from build123d import *

# Parameters (mm, degrees)
SKETCH2_R           = 55
BOSS_EXTRUDE1_DEPTH = 70
SHELL1_T            = -5
SKETCH4_R           = 125
BOSS_EXTRUDE2_DEPTH = 1
RIB7_REACH          = 192.132
SKETCH3_WALL_W      = 472.644862012
SKETCH3_WALL_H      = 10
CIRPATTERN1_COUNT   = 4
CUT_EXTRUDE1_DEPTH  = 1
CIRPATTERN2_COUNT   = 4
CUT_EXTRUDE2_DEPTH  = 194.455421222
CIRPATTERN3_COUNT   = 4
SKETCH10_W          = 64.387061578
SKETCH10_H          = 55
CUT_EXTRUDE3_DEPTH  = 191.131533418
CIRPATTERN4_COUNT   = 2
CIRPATTERN4_ANGLE   = 90


with BuildPart() as part:
    # Sketch2 → Boss-Extrude1 (new body)
    with BuildSketch(Plane(origin=(0, 0, 0), x_dir=(1, 0, 0), z_dir=(0, 1, 0))):
        with Locations(Location((0, 0, 0), (0, 0, 270))):
            Circle(SKETCH2_R)
    extrude(amount=BOSS_EXTRUDE1_DEPTH)

    # Shell1
    shell1_openings = [part.faces().sort_by_distance(p)[0] for p in [
        (0, 70, 0),
    ]]
    offset(amount=SHELL1_T, openings=shell1_openings, kind=Kind.INTERSECTION)

    # Sketch4 → Boss-Extrude2 (add)
    with BuildSketch(Plane(origin=(0, 0, 0), x_dir=(1, 0, 0), z_dir=(0, 1, 0))):
        with Locations(Location((0, 0, 0), (0, 0, 270))):
            Circle(SKETCH4_R)
    extrude(amount=BOSS_EXTRUDE2_DEPTH)

    # Sketch3 wall → Rib7 (add, up to next)
    with BuildSketch(Plane(origin=(87, 32.90951621, 0), x_dir=(0.708107200971, -0.706104943994, 0), z_dir=(0.706104943994, 0.708107200971, 0)), mode=Mode.PRIVATE) as rib7_sk1:
        Rectangle(SKETCH3_WALL_W, SKETCH3_WALL_H)
    rib7_tool1 = extrude(rib7_sk1.sketch, amount=-RIB7_REACH, mode=Mode.PRIVATE) - part.part
    rib7 = rib7_tool1.solids().sort_by_distance((87, 32.90951621, 0))[0]
    add(rib7)

    # CirPattern1: Rib7 ×4 about axis
    cirpattern1_axis = Axis((0, 0, 0), (0, 1, 0))
    for i in range(1, CIRPATTERN1_COUNT):
        add(rib7.rotate(cirpattern1_axis, i * 360 / CIRPATTERN1_COUNT))

    # Sketch5 → Cut-Extrude1 (cut)
    with BuildSketch(Plane(origin=(0, 1, 0), x_dir=(1, 0, 0), z_dir=(0, 1, 0))):
        with BuildLine():
            Line((9.493142678, -59.24424227), (9.493142678, -129.652922227))
            ThreePointArc((9.493142678, -129.652922227), (92.201319164, -91.645604065), (129.707942461, -8.709171177))
            Line((129.707942461, -8.709171177), (59.364554554, -8.709171177))
            ThreePointArc((59.364554554, -8.709171177), (42.705900876, -42.145059383), (9.493142678, -59.24424227))
        make_face()
    cut_extrude1 = extrude(amount=-CUT_EXTRUDE1_DEPTH, mode=Mode.SUBTRACT)

    # CirPattern2: Cut-Extrude1 ×4 about axis
    cirpattern2_axis = Axis((0, 0, 0), (0, 1, 0))
    for i in range(1, CIRPATTERN2_COUNT):
        add(cut_extrude1.rotate(cirpattern2_axis, i * 360 / CIRPATTERN2_COUNT), mode=Mode.SUBTRACT)

    # Sketch7 → Cut-Extrude2 (cut, through all)
    with BuildSketch(Plane(origin=(5, 0, 0), x_dir=(0, 0, -1), z_dir=(1, 0, 0))):
        Polygon((59.772255751, 52.99919304), (106.904721419, 6), (59.772255751, 6), align=None)
    cut_extrude2 = extrude(amount=-CUT_EXTRUDE2_DEPTH, mode=Mode.SUBTRACT)

    # CirPattern3: Cut-Extrude2 ×4 about axis
    cirpattern3_axis = Axis((0, 0, 0), (0, 1, 0))
    for i in range(1, CIRPATTERN3_COUNT):
        add(cut_extrude2.rotate(cirpattern3_axis, i * 360 / CIRPATTERN3_COUNT), mode=Mode.SUBTRACT)

    # Sketch10 → Cut-Extrude3 (cut, symmetric)
    with BuildSketch(Plane(origin=(0, 0, 0), x_dir=(0.7117650145966598, -3.2873850610052313e-15, 0.7024176563813135), z_dir=(-0.7024176563813135, -3.331131634682351e-15, 0.7117650145966598))):
        with Locations((-0.279356343, 36.5)):
            Rectangle(SKETCH10_W, SKETCH10_H)
    cut_extrude3 = extrude(amount=CUT_EXTRUDE3_DEPTH, both=True, mode=Mode.SUBTRACT)

    # CirPattern4: Cut-Extrude3 ×2 about axis
    cirpattern4_axis = Axis((0, 70, 0), (0, 1, 0))
    for i in range(1, CIRPATTERN4_COUNT):
        add(cut_extrude3.rotate(cirpattern4_axis, i * CIRPATTERN4_ANGLE / (CIRPATTERN4_COUNT - 1)), mode=Mode.SUBTRACT)


solid = part.part
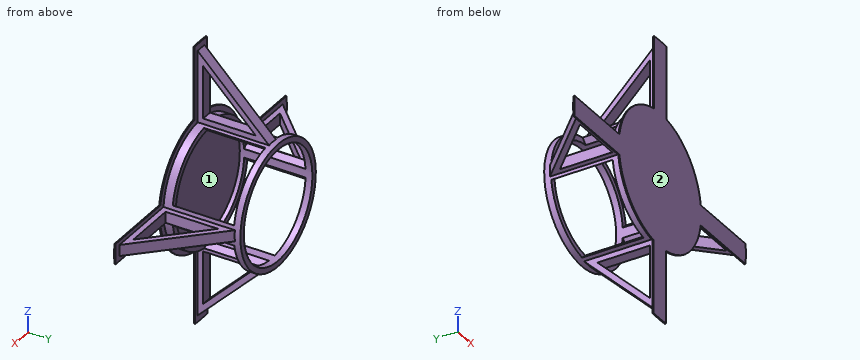
Input: part model. Units: mm. Frame: model coordinates. Face numbers are marked on the shaded views. Coordinates: 2 decimals unless noted, no trailing zeros. Loops run counter-clockwise (first coordinate to the right, second up) from the corner with the lowest first, then second, coordinate; pieces in that order, holes last. Notation, with made-up numbers: (-20.5, -31.5) -> (11.5, -31.5) arc R33 cw to (11.5, 4.5) -> close; hole circle Ø2 at (-23.75, 69.5). An arc over 180 degrees is marked (long way). Write item = value, one per line. Start each with the question number.
Item 1: Mould query, pull axis Z, two halves, no side actions, for the marked faces 1 and 2. Classes: pulls with the +Z half, pulls with the -Z half, needs draft (parallel to the pull), parting line crosses it, or undercut.
Item 2: Cut plane D-D, the plane x = 74.5. Return loops of the section in (y, z), plus the area to 3 significant figures.
Item 3: First-contact query: P1, Ø0.8, axis at y = 0.5, z = -104, coming from the +X side; P2, Ø8, axis at y = 32, z = 3, coming from the +X side; P3, Ø8, axis at x = 0.5, z = -94, coming from the +Y side; P4, Ø12, axis at x = -88, y = 41.5, coming from the -Z side. Flat tips, straight axial feed; report the tip coordinate or a pass-through.
Item 4: Cut plane C-C, the plane y = 60. Count the separate pieces of the cut face and the enclosed holes in it, plus the area to 3 significant figures.
Item 5: Cut plane A-A, the plane z = 26. Return loops of the section in (x, y), plus the area to 3 significant figures.
Item 6: Material intervals for line 1 (X direction, y = 27.5, z = 0); line 2 (Z direction, x = 0, y = 25); line 3 (Z direction, x = 0, y = 28), sorted ascending.
Item 7: Cut plane B-B, the plane x = 18.5. Return loops of the section in (y, z), plus the area to 3 significant figures.
Ans:
q1.face_1 = undercut
q1.face_2 = needs draft
q2.outline = (0, -9.49) -> (1, -9.49) -> (1, -5) -> (6, -5) -> (6, 5) -> (1, 5) -> (1, 8.71) -> (0, 8.71) -> close; (38.31, -5) -> (45.37, -5) -> (45.37, 5) -> (38.31, 5) -> close
q2.area = 139 mm²
q3.P1 = 8.71
q3.P2 = 91.92
q3.P3 = 29.92
q3.P4 = through
q4.separate_pieces = 4
q4.enclosed_holes = 0
q4.area = 459 mm²
q5.outline = (-54.07, 0) -> (54.07, 0) -> (54.07, 1) -> (48.47, 1) -> (48.47, 9) -> (42.71, 9) -> (42.71, 5) -> (-42.71, 5) -> (-42.71, 9) -> (-48.47, 9) -> (-48.47, 1) -> (-54.07, 1) -> close; (-48.47, 64) -> (-42.71, 64) -> (-42.71, 70) -> (-48.47, 70) -> close; (42.71, 64) -> (48.47, 64) -> (48.47, 70) -> (42.71, 70) -> close
q5.area = 611 mm²
q6.line_1 = -92.42 to -85.34, -59.77 to -50, 50 to 59.77, 85.34 to 92.42
q6.line_2 = -94.93 to -87.85, -59.77 to -50, 50 to 59.77, 87.85 to 94.93
q6.line_3 = -91.92 to -84.84, -59.77 to -50, 50 to 59.77, 84.84 to 91.92
q7.outline = (0, -57.08) -> (1, -57.08) -> (1, -51.8) -> (9, -51.8) -> (9, -46.45) -> (5, -46.45) -> (5, 46.45) -> (9, 46.45) -> (9, 51.8) -> (1, 51.8) -> (1, 57.08) -> (0, 57.08) -> close; (64, -51.8) -> (70, -51.8) -> (70, -46.45) -> (64, -46.45) -> close; (64, 46.45) -> (70, 46.45) -> (70, 51.8) -> (64, 51.8) -> close
q7.area = 635 mm²
